```python
from build123d import *

# Parameters (mm, degrees)
BOSS_EXTRUDE1_DEPTH = 50
SKETCH4_R           = 7.5
CUT_EXTRUDE1_DEPTH  = 30
SKETCH5_R           = 4.5
CUT_EXTRUDE2_DEPTH  = 26.46703487


with BuildPart() as part:
    # Sketch2 → Boss-Extrude1 (new body)
    with BuildSketch(Plane(origin=(0, 0, 0), x_dir=(1, 0, 0), z_dir=(0, 1, 0))):
        Polygon((3.535533906, 22.535533906), (3.535533906, 7.535533906), (0, 11.071067812), (0, 0), (30, 0), (30, 30), (0, 30), (0, 19), align=None)
    extrude(amount=BOSS_EXTRUDE1_DEPTH)

    # Sketch4 → Cut-Extrude1 (cut)
    with BuildSketch(Plane(origin=(12.477367975, 54.045418359, 0), x_dir=(0, 0, -1), z_dir=(0.224951054, 0.974370065, 0))):
        with Locations((13, -1.197365684)):
            Circle(SKETCH4_R)
    extrude(amount=-CUT_EXTRUDE1_DEPTH, mode=Mode.SUBTRACT)

    # Sketch5 → Cut-Extrude2 (cut, through all)
    with BuildSketch(Plane(origin=(5.728836345, 24.814316416, 0), x_dir=(0.974370065, -0.224951054, 0), z_dir=(0.224951054, 0.974370065, 0))):
        with Locations((1.197365684, 13)):
            Circle(SKETCH5_R)
    extrude(amount=-CUT_EXTRUDE2_DEPTH, mode=Mode.SUBTRACT)


solid = part.part
```
Verification items for the finished model (mm, model axes). A direction names the side the tool comes from. Give positions to 0.01 mm unless a question says otherwise; leave off trailing zeros. Loops run counter-clockwise (first coordinate to the right, second up) from the corner with the lowest first, then second, coordinate; pieces in that order, holes last.
1. Section check A-A, the plane z = -14. Enter the section's corners in (x, y).
2. Go/stop test with a flat-tipped pin: pin 1 Ø4 at (x, z) = (7.5, -6.5) entering from -Y. Record where the tip stops, or that it passes through.
3. Section check B-B, the plane z = -6.25. Enter the section's corners in (x, y).
4. Thickness scan on line 1 (Z direction, x = 9.5, y = 35); line 2 (X direction, y = 32, z = -19.25); line 3 (Z direction, x = 7.5, y = 39). Record the ranges inside material, lowest first.
5. Set-up check for faces 1 (the flat face through (2, 25, -21)), 2 (the cylindrical face through (0.985, 7.523, -8.935)), 3 (the flat face through (15, 0, -15)): record each of +Z, -Z, +X, -X, +Y, -Y from which the full face is reachable in a straight line by a thin tool's end or side.
6. Mould release check, pull along Z, two halves, no side actions. Record for faces 4 (the cylindrical face through (17.21, 36.68, -11.37)), 5 (the flat face through (15, 25, -30)), 6 (the flat face through (0, 25, -6)): released by +Z, released by -Z, zero draft, split by the parting line, or undercut.
Geometry says:
1. outline: (3.54, 43.03) - (5.14, 50) - (3.54, 50) - close; (5.73, 0) - (30, 0) - (30, 50) - (20.4, 50) - (14.14, 22.87) - (11.17, 23.56) - close
2. pin 1: stops at y = 0
3. outline: (0, 0) - (30, 0) - (30, 50) - (16.13, 50) - (10.08, 23.81) - (3.71, 25.28) - (9.42, 50) - (0, 50) - close
4. line 1: z = -30 to -20.5, -5.5 to 0
4. line 2: x = 0 to 0.25, 3.54 to 4.36, 12.87 to 30
4. line 3: z = -30 to -20.01, -5.99 to 0
5. face 1: +Y, -Y
5. face 2: none
5. face 3: +Z, -Z, +X, -X, -Y
6. face 4: undercut
6. face 5: released by -Z
6. face 6: zero draft
